The listing builds one solid part. Answer for the finished solid, in the listing's coordinates (mm). A direction names the side the tool comes from. Round coordinates to 2 decimals unless told otherwise and drop trailing zeros. Loops run counter-clockwise (first coordinate to the right, second up) from the corner with the lowest first, then second, coordinate; pieces in that order, holes last. Notation, with made-up numbers: (70.25, 46.5) - (103.25, 46.5) arc R19 cw to (103.25, 55.5) - close; hole circle Ø11 at (-12.75, 59.5). An arc over 180 degrees is marked (long way). Write item = value, one per line. Start each with the question number.
1) For a pull along Z with two mould halves and no side action, classify faces 4 (the cylindrical face through (-2.17, 29.58, -9.76)), 5 (the flat face through (-3.8, 80, -7.3)), 6 (the flat face through (3.944, 74.084, -6.961)) as released by +Z, released by -Z, zero draft, split by the parting line, or undercut.
2) Section D-D, the plane y = 35.5 is taken. Determine the outline of the cut face in (x, z), and give its area (3 significant figures).
3) Section A-A, the plane y = 69.5 is taken. Determine the outline of the cut face in (x, z), and give its area (3 significant figures).
4) A tool of negligible diameter and unlimited length cuts with its end or side. For faces 1 (the flat face through (-0.2, 60, 10.4)), 2 (the flat face through (8, 74, 0)), 3 (the flat face through (0, 0, 0)), from which of +Z, -Z, +X, -X, +Y, -Y can it reach the whole face along a straight path? Write none if from no direction.
5) Section C-C, the plane x = 5.5 is taken. Determine the outline of the cut face in (y, z), and give its area (3 significant figures).
6) Section B-B, the plane z = 0 is taken. Determine the outline of the cut face in (x, y).
7) Given pin 1 Ø4 at (x, z) = (-3, 2.5) entering from +Y; pin 2 Ø5 at (y, z) = (54.5, -11) entering from -X; pin 3 Ø10 at (x, y) = (9.5, 35.5) entering from -Z, each flat-ended and moving along its own axis, determine where each tip first touches the part or whether it passes through.
8) Straight lines are drawn through the part: line 1 along Y through (x, z) = (-3.5, -12.5); line 2 along Y through (x, z) = (1, -8); line 3 along Z through (x, y) = (3, 54.5). For each, find the intervals that lie inside material, in ascending order.
Autodesk Inventor part; units mm, degrees
ref_plane "YZ Plane" through (0, 0, 0) normal (1, 0, 0) x (0, 1, 0)
ref_plane "XZ Plane" through (0, 0, 0) normal (0, 1, 0) x (-1, 0, 0)
ref_plane "XY Plane" through (0, 0, 0) normal (0, 0, 1) x (1, 0, 0)
sketch "Sketch1" plane through (0, 0, 0) normal (0, 0, 1) x (1, 0, 0)
  line L0 (0, 0) -> (0, 80)
  line L1 (0, 80) -> (16, 80)
  line L2 (16, 80) -> (16, 60)
  line L3 (16, 60) -> (10, 60)
  line L4 (10, 60) -> (10, 0)
  line L5 (0, 0) -> (10, 0)
  dimension "d" = 20
  dimension "HT" = 20
  dimension "Height" = 60
  dimension "HD" = 32
revolve "Revolution1" add sketch "Sketch1" angle 360 about axis through (0, 0, 0) along (0, 1, 0)
sketch "Sketch2" plane through (0, 80, 0) normal (0, 1, 0) x (1, 0, 0)
  line L0 (0, 9.2376) -> (8, 4.6188)
  line L1 (8, 4.6188) -> (8, -4.6188)
  line L2 (8, -4.6188) -> (0, -9.2376)
  line L3 (0, -9.2376) -> (-8, -4.6188)
  line L4 (-8, -4.6188) -> (-8, 4.6188)
  line L5 (-8, 4.6188) -> (0, 9.2376)
  point P0 (0, 0)
  point P1 (0, 0)
  dimension "HL" = 16
extrude "Extrusion1" cut sketch "Sketch2" against normal blind 12
equation "\"HT\" = d"
equation "\"Height\" = 3 * d"
equation "\"HD\" = 1.6 * d"
equation "\"HL\" = 0.8 * d"
equation "\"HH\" = 0.6 * d"
properties part number "CE-2.1.5-01"
Geometry check:
q1.face_4 = split by the parting line
q1.face_5 = zero draft
q1.face_6 = undercut
q2.outline = circle Ø20 at (0, 0)
q2.area = 314 mm2
q3.outline = circle Ø32 at (0, 0); hole (-8, -4.62) - (0, -9.24) - (8, -4.62) - (8, 4.62) - (0, 9.24) - (-8, 4.62) - close
q3.area = 583 mm2
q4.face_1 = -Y
q4.face_2 = +Y
q4.face_3 = +Z, -Z, +X, -X, -Y
q5.outline = (0, -8.35) - (60, -8.35) - (60, -15.02) - (80, -15.02) - (80, -6.06) - (68, -6.06) - (68, 6.06) - (80, 6.06) - (80, 15.02) - (60, 15.02) - (60, 8.35) - (0, 8.35) - close
q5.area = 1,460 mm2
q6.outline = (-16, 60) - (-10, 60) - (-10, 0) - (10, 0) - (10, 60) - (16, 60) - (16, 80) - (8, 80) - (8, 68) - (-8, 68) - (-8, 80) - (-16, 80) - close
q7.pin_1 = 68
q7.pin_2 = -5.27
q7.pin_3 = -8.93
q8.line_1 = 60 to 80
q8.line_2 = 0 to 68
q8.line_3 = -9.54 to 9.54
